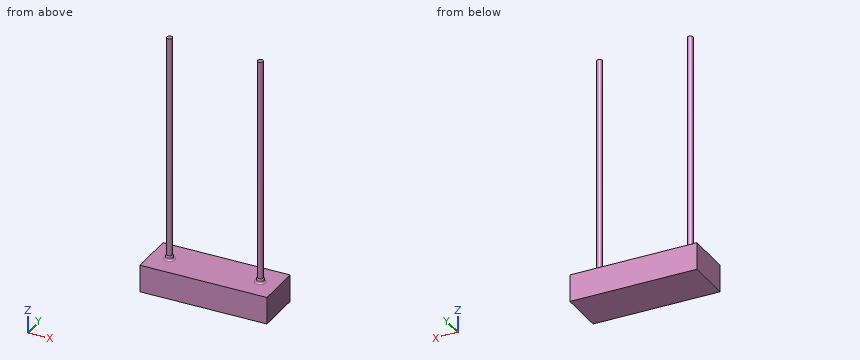
Autodesk Inventor part; units mm, degrees
ref_plane "YZ Plane" through (0, 0, 0) normal (1, 0, 0) x (0, 1, 0)
ref_plane "XZ Plane" through (0, 0, 0) normal (0, 1, 0) x (-1, 0, 0)
ref_plane "XY Plane" through (0, 0, 0) normal (0, 0, 1) x (1, 0, 0)
sketch "Sketch1" plane through (0, 0, 0) normal (0, 0, 1) x (1, 0, 0)
  line L0 (0, 0) -> (14, 0)
  line L1 (14, 0) -> (14, 5)
  line L2 (14, 5) -> (0, 5)
  line L3 (0, 5) -> (0, 0)
  dimension "d39" = 14
  dimension "d40" = 5
extrude "Extrusion1" add sketch "Sketch1" along normal mid plane 3
ref_plane "Work Plane5" through (0, 0, 1.5) normal (0, 0, 1) x (1, 0, 0)
sketch "Sketch9" plane through (0, 0, 1.5) normal (0, 0, 1) x (1, 0, 0)
  line L0 (0, 5) -> (0, 0)
  line L1 (0, 2.5) -> (2, 2.5)
  line L2 (14, 0) -> (14, 5)
  line L3 (14, 2.5) -> (12, 2.5)
  circle A0 centre (12, 2.5) radius 0.4
  circle A1 centre (2, 2.5) radius 0.4
  dimension "d43" = 2
  dimension "d44" = 2
  dimension "d45" = 0.8
  dimension "d46" = 0.8
extrude "Extrusion5" add sketch "Sketch9" along normal blind 0.5
fillet "Fillet5" radius 0.2 4 edges at (11.6, 2.5, 1.5) (11.6, 2.5, 2) (1.6, 2.5, 1.5) (1.6, 2.5, 2)
sketch "Sketch10" plane through (14, 0, 1.5) normal (1, 0, 0) x (0, 0, -1)
  line L0 (3, 5) -> (3, 0)
  line L1 (3, 2.5) -> (0, 2.5)
  line L2 (0, 0) -> (0, 5)
  point P0 (1.5, 0)
sketch "Sketch11" plane through (0, 0, 1.5) normal (0, 0, 1) x (1, 0, 0)
  line L0 (14, 0) -> (14, 5)
  circle A0 centre (12, 2.5) radius 0.2
  line L1 (7.4995, 2.5) -> (3.1588, 2.5)
  point P0 (0, 0)
sketch "Sketch12" plane through (0, 0, 1.5) normal (-1, 0, 0) x (0, 0, 1)
  line L0 (-3, 5) -> (-3, 0)
  line L1 (-3, 2.5) -> (0, 2.5)
  line L2 (0, 1.9) -> (0, 3.1)
  point P0 (-1.5, 0)
sketch "Sketch13" plane through (0, 0, 1.5) normal (0, 0, 1) x (1, 0, 0)
  line L0 (0, 5) -> (0, 0)
  point P0 (0, 2.5)
ref_plane "Work Plane7" through (2, 2.5, 2) normal (0, 0, 1) x (1, 0, 0)
ref_plane "Work Plane8" through (12, 2.5, 2) normal (0, 0, 1) x (1, 0, 0)
sketch "Sketch15" plane through (2, 2.5, 2) normal (0, 0, 1) x (1, 0, 0)
  circle A0 centre (0, 0) radius 0.2
  circle A1 centre (0, 0) radius 0.3
  point P0 (-2, -2.5)
  dimension "d57" = 0.6
sketch "Sketch17" plane through (12, 2.5, 2) normal (0, 0, 1) x (1, 0, 0)
  circle A0 centre (0, 0) radius 0.3
  point P0 (-12, -2.5)
  dimension "d63" = 0.6
ref_plane "Work Plane9" through (0, 2.5, -1.5) normal (0, -1, 0) x (0, 0, 1)
sketch "Sketch18" plane through (0, 2.5, -1.5) normal (0, -1, 0) x (0, 0, 1)
  line L0 (3, -2) -> (28, -2)
  line L1 (2.9646, -12) -> (27.9646, -12)
  point P0 (1.5, 0)
  point P1 (3, 0)
  dimension "d66" = 2
  dimension "d67" = 25
  dimension "d69" = 25
sweep "Sweep6" add profiles "Sketch15" path "Sketch18" path curves L0 contours A0 | A1
sweep "Sweep7" add profiles "Sketch17" path "Sketch18" path curves L1
equation "\"BendRadius\" = Thickness"
equation "\"BendReliefWidth\" = Thickness"
equation "\"BendReliefDepth\" = 0.5 * Thickness"
equation "\"CornerReliefSize\" = 4 * Thickness"
equation "\"MinimumRemnant\" = 2 * Thickness"
equation "\"TransitionRadius\" = BendRadius"
equation "\"JacobiRadiusSize\" = BendRadius"
equation "\"GapSize\" = Thickness"
properties part number "A54"
Build history of the part. All positions in model axes, mm. Round coordinates to 2 decimals unless told otherwise and drop trailing zeros. Write each loop counter-clockwise with the first axis right and the second up, starting at its lowest first coordinate (ties: lowest second). Pieces come first, ordered by that corner, then holes. Notation, with made-up numbers: (59, 34) - (114, 34) arc R22 ccw to (114, 43) - close; hole circle Ø1 at (35.5, 12.5). An arc over 180 degrees is marked (long way). Write each question's results on one line, items separated by ' | '. Start each with the question number.
Item 1: Saw through at A-A (z = 11.75). Write the cut outline in (x, y).
Item 2: Wall check: L1, parallel to Y at x = 2, z = 14.75; L2, parallel to Z at x = 8, y = 4.05; L3, parallel to X at y = 2.35, z = 11. Give the ranges that are in metal, low to high. Write a range as [from, to].
Item 3: Saw through at B-B (x = 7.5). Write the cut outline in (y, z), and give its area (3 significant figures).
Item 4: Saw through at C-C (y = 1). Write the cut outline in (x, z), and give its area (3 significant figures).
Item 5: Drop flat-ended pins along their axis: P1, Ø0.7, axis at x = 12, y = 2.5, coming from the +Z side; P2, Ø1, axis at x = 2, y = 1, coming from the +Z side; P3, Ø4, axis at x = 10, z = 15.5, coming from the +Y side. Give the stop position or say it passes through.
Results are:
1) outline: circle Ø0.6 at (2, 2.5); circle Ø0.6 at (12, 2.5)
2) L1: y = [2.2, 2.8] | L2: z = [-1.5, 1.5] | L3: x = [1.74, 2.26], [11.74, 12.26]
3) outline: (0, -1.5) - (5, -1.5) - (5, 1.5) - (0, 1.5) - close | area: 15.0 mm²
4) outline: (0, -1.5) - (14, -1.5) - (14, 1.5) - (0, 1.5) - close | area: 42.0 mm²
5) P1: stops at z = 26.46 | P2: stops at z = 1.5 | P3: stops at y = 2.8
